```python
from build123d import *

# Parameters (mm, degrees)
F0_W     = 1066.8
F0_H     = 342.9
F1_DEPTH = 50.8
F2_R     = 38.1
F3_W     = 41.275
F3_H     = 88.9
F4_DEPTH = 50.8
F7_DEPTH = 50.8
F8_DEPTH = 50.8


with BuildPart() as f1:
    # F0 (on Top) → F1 (new body)
    with BuildSketch(Plane.XY):
        Rectangle(F0_W, F0_H)
    extrude(amount=F1_DEPTH)

    # F2
    f2_edges = [f1.edges().sort_by_distance(p)[0] for p in [
        (-533.4, 171.45, 25.4),
        (-533.4, -171.45, 25.4),
        (533.4, 171.45, 25.4),
        (533.4, -171.45, 25.4),
    ]]
    fillet(f2_edges, radius=F2_R)

    # F3 (on face) → F4 (cut)
    with BuildSketch(Plane.XY.offset(50.8)):
        with Locations((512.7625, 127)):
            Rectangle(F3_W, F3_H)
        with Locations((512.7625, -127)):
            Rectangle(F3_W, F3_H)
    extrude(amount=-F4_DEPTH, mode=Mode.SUBTRACT)

    # F6 (on face) → F7 (cut)
    with BuildSketch(Plane.XY.offset(50.8)):
        with BuildLine():
            ThreePointArc((-279.4, 44.45127), (-234.95, 0.00127), (-190.5, 44.45127))
            ThreePointArc((-190.5, 44.45127), (-190.854197, 50.05151), (-191.911145, 55.5625))
            ThreePointArc((-191.911145, 55.5625), (-240.55024, 88.547073), (-279.4, 44.45127))
        make_face()
        with BuildLine():
            ThreePointArc((-191.911145, 55.5625), (-190.854197, 50.05151), (-190.5, 44.45127))
            ThreePointArc((-190.5, 44.45127), (-234.95, 0.00127), (-279.4, 44.45127))
            Line((-279.4, 44.45127), (-279.4, -44.45127))
            ThreePointArc((-279.4, -44.45127), (-234.95, -0.00127), (-190.5, -44.45127))
            ThreePointArc((-190.5, -44.45127), (-190.854197, -50.05151), (-191.911145, -55.5625))
            Line((-191.911145, -55.5625), (263.731644, -55.5625))
            Line((263.731644, -55.5625), (285.221681, -87.023401))
            Line((285.221681, -87.023401), (342.9, -47.625))
            Line((342.9, -47.625), (438.15, -47.625))
            Line((438.15, -47.625), (438.15, 41.275))
            Line((438.15, 41.275), (396.875, 41.275))
            ThreePointArc((396.875, 41.275), (372.479858, 66.485039), (342.9, 47.625))
            Line((342.9, 47.625), (285.221681, 87.023401))
            Line((285.221681, 87.023401), (263.731644, 55.5625))
            Line((263.731644, 55.5625), (-191.911145, 55.5625))
        make_face()
        with BuildLine():
            ThreePointArc((-190.5, -44.45127), (-234.95, -0.00127), (-279.4, -44.45127))
            ThreePointArc((-279.4, -44.45127), (-240.55024, -88.547073), (-191.911145, -55.5625))
            ThreePointArc((-191.911145, -55.5625), (-190.854197, -50.05151), (-190.5, -44.45127))
        make_face()
    extrude(amount=-F7_DEPTH, mode=Mode.SUBTRACT)

    # F5 (on face) → F8 (cut)
    with BuildSketch(Plane.XY.offset(50.8)):
        Polygon((-400.05, 47.625), (-457.2, 47.625), (-457.2, -47.625), (-400.05, -47.625), (-400.05, -15.875), (-330.2, -15.875), (-330.2, 15.875), (-400.05, 15.875), align=None)
    extrude(amount=-F8_DEPTH, mode=Mode.SUBTRACT)


solid = f1.part
```
Model file for the job. Use its own axes, mm. A direction names the side the tool comes from. Coordinates: 2 decimals unless noted, no trailing zeros. Loops run counter-clockwise (first coordinate to the right, second up) from the corner with the lowest first, then second, coordinate; pieces in that order, holes last. Notation, with made-up numbers: M 28.5,27.25 L 71.5,27.25 A5 cw 71.5,35.25 Z; hole C 62.25,-32 d6. An arc over 180 degrees is marked long. Use CSV: the item, a comma, the result in double quotes. Start each with the question number.
1. Two-plate mould, pull along Y, no slides. Class faces 1 (the flat face through (-8, 171.45, 25)), 2 (the flat face through (-8, -171.45, 25)), 3 (the cylindrical face through (-239.66, 88.65, 25.76)), 4 (the flat face through (-533.4, -2, 25)): pulls with the +Y half, pulls with the -Y half, needs draft (parallel to the pull), parting line crosses it, or undercut.
2. Band-saw the part on A-A, the plane x = -129.5. List the corners of the cut face in (y, z).
3. Probe probe 1 along X at (y, z) = (-41, 27.5); probe 2 along X at (y, z) = (-3, 41); probe 3 along Y at (x, z) = (-343, 4) (3 decimals). List the from-to ranges inside material, lowest first. Write a range as [from, to].
4. Tool access for faces 5 (the flat face through (492.125, -128, 26)), 6 (the flat face through (492.125, 126, 26)), 7 (the flat face through (39, 55.562, 26)): list every direction of +Z, -Z, +X, -X, +Y, -Y with a clear straight run to the whole face (end or side of a thin tool).
5. Band-saw the part on B-B, the plane y = -32.5. List the corners of the cut face in (x, z).
6. Band-saw the part on C-C, the plane z = 39. Give the number of separate pieces and of enclosed holes in the cut face, then the cut area to 3 significant figures.
7. Flat gauge pins, fed straight in: pin 1 (12.5 mm diameter, centred on x = 506.5, z = 33, fed in from +Y); pin 2 (8 mm diameter, centred on y = 86.5, z = 37.5, fed in from +X). Where does each tip first touch, or does it go through?
8. Band-saw the part on D-D, the plane y = 146.5. List the corners of the cut face in (x, z) (3 decimals), then the cut area to 3 significant figures.
Entries:
1,face 1,"pulls with the +Y half"
1,face 2,"pulls with the -Y half"
1,face 3,"undercut"
1,face 4,"needs draft"
2,outline,"M -171.45,0 L -55.56,0 L -55.56,50.8 L -171.45,50.8 Z; M 55.56,0 L 171.45,0 L 171.45,50.8 L 55.56,50.8 Z"
3,probe 1,"x = [-533.4, -457.2], [-400.05, -279.4], [438.15, 533.4]"
3,probe 2,"x = [-533.4, -457.2], [-330.2, -279.4], [438.15, 533.4]"
3,probe 3,"y = [-171.45, -15.875], [15.875, 171.45]"
4,face 5,"+Z, -Z, +X, -Y"
4,face 6,"+Z, -Z, +X, +Y"
4,face 7,"+Z, -Z"
5,outline,"M -533.4,0 L -457.2,0 L -457.2,50.8 L -533.4,50.8 Z; M -400.05,0 L -279.4,0 L -279.4,50.8 L -400.05,50.8 Z; M 438.15,0 L 533.4,0 L 533.4,50.8 L 438.15,50.8 Z"
6,separate pieces,"1"
6,enclosed holes,"2"
6,area,"265,000 mm2"
7,pin 1,"stops at y = 82.55"
7,pin 2,"stops at x = 533.4"
8,outline,"M -531.059,0 L 492.125,0 L 492.125,50.8 L -531.059,50.8 Z"
8,area,"52,000 mm2"
